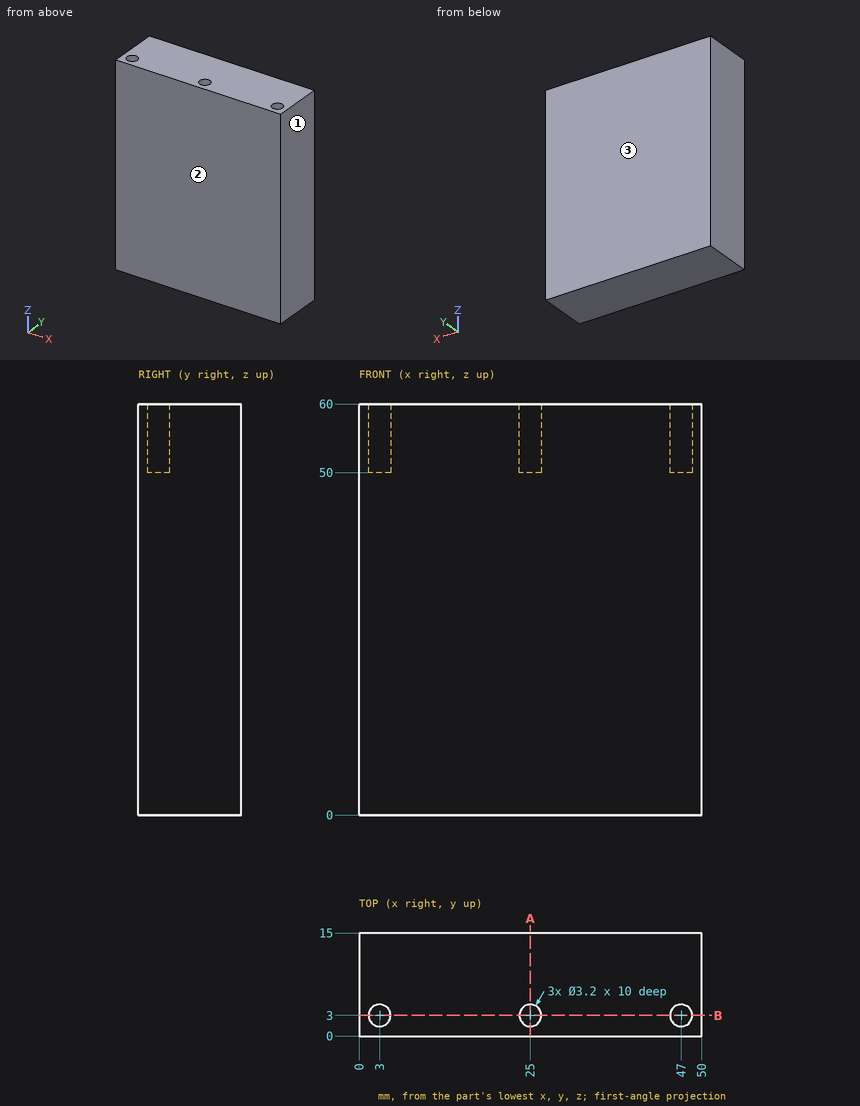
Answer from the drawing. Dimensions are ordinates in mm from the lowest x, y and z of the part. Round coordinates to 2 decimals unless told otherwise and drop trailing zeros. Loops run counter-clockwise (first coordinate to the right, second up) from the corner with the lowest first, then second, coordinate; pieces in that order, holes last.
(1) This flat-tipped pin is pushed along its axis until it touches: P1, Ø2.5, axis at x = 47, y = 3, coming from the +Z side. Where does it stop, or does it pass through?
Computed values:
P1: stops at z = 50
(2) The part is cut by section B-B, the plane y = 3. Give the vertices of the cut face in (x, z), and give its area (3 significant figures).
Computed values:
outline: (0, 0) - (50, 0) - (50, 60) - (48.6, 60) - (48.6, 50) - (45.4, 50) - (45.4, 60) - (26.6, 60) - (26.6, 50) - (23.4, 50) - (23.4, 60) - (4.6, 60) - (4.6, 50) - (1.4, 50) - (1.4, 60) - (0, 60) - close
area: 2,900 mm2
(3) The part is cut by section A-A, the plane x = 25. Give the vertices of the cut face in (y, z), and give its area (3 significant figures).
Computed values:
outline: (0, 0) - (15, 0) - (15, 60) - (4.6, 60) - (4.6, 50) - (1.4, 50) - (1.4, 60) - (0, 60) - close
area: 868 mm2
(4) Find the intervals of material crossed by L1, parallel to Y at x = 25, z = 55; L2, parallel to Z at x = 4, y = 3.25, in increasing order.
Computed values:
L1: y = 0 to 1.4, 4.6 to 15
L2: z = 0 to 50
(5) The mould has two halves that part along Y. Classify the marked faces 1, 2 and 3: pulls with the +Y half, pulls with the -Y half, needs draft (parallel to the pull), parting line crosses it, or undercut.
Computed values:
face 1: needs draft
face 2: pulls with the -Y half
face 3: pulls with the +Y half
